from build123d import *

# Parameters (mm, degrees)
F0_R     = 5.08
F1_DEPTH = 91.44
F2_R     = 0.99
F3_DEPTH = 88.9
F4_SIZE  = 2.54
F5_R     = 5.08


with BuildPart() as f1:
    # F0 (on Front) → F1 (new body)
    with BuildSketch(Plane.XZ):
        Circle(F0_R)
    extrude(amount=F1_DEPTH)

    # F2 (on face) → F3 (cut)
    with BuildSketch(Plane.XZ.offset(91.44)):
        Circle(F2_R)
    extrude(amount=-F3_DEPTH, mode=Mode.SUBTRACT)

    # F4
    f4_edges = [f1.edges().sort_by_distance(p)[0] for p in [
        (-5.08, -91.44, 0),
    ]]
    chamfer(f4_edges, length=F4_SIZE)

    # F5
    f5_edges = [f1.edges().sort_by_distance(p)[0] for p in [
        (-5.08, 0, 0),
    ]]
    fillet(f5_edges, radius=F5_R)


solid = f1.part
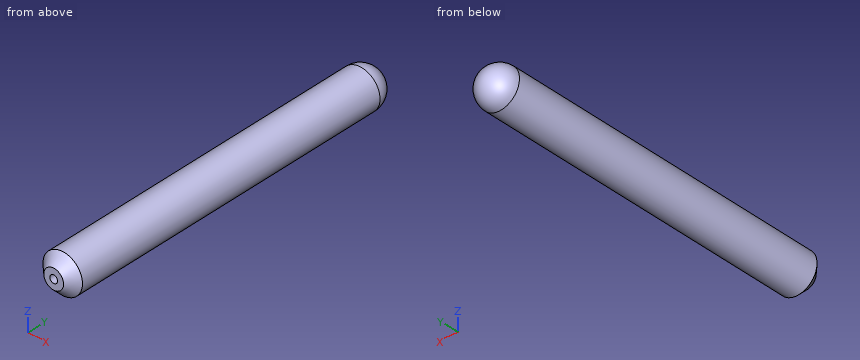
The listing builds one solid part. Answer for the finished solid, in the listing's coordinates (mm). Give positions to 0.01 mm unless a question says otherwise; leave off trailing zeros. Write each loop counter-clockwise with the first axis right and the second up, starting at its lowest first coordinate (ties: lowest second). Pieces come first, ordered by that corner, then holes. Notation, with made-up numbers: (-19.75, -16) -> (28.25, -16) arc R22 cw to (28.25, 17) -> close; hole circle Ø3 at (22.5, -24). An arc over 180 degrees is marked (long way). Use a Markdown table: item, result.
(1) Section A-A, the plane x = 0 is taken. Determine the outline of the cut face in (y, z).
Return value:
| item | result |
|---|---|
| outline | (-91.44, -2.54) -> (-88.9, -5.08) -> (-5.08, -5.08) arc R5.08 ccw to (-5.08, 5.08) -> (-88.9, 5.08) -> (-91.44, 2.54) -> (-91.44, 0.99) -> (-2.54, 0.99) -> (-2.54, -0.99) -> (-91.44, -0.99) -> close |
(2) Flat-ended cylindrical pins translate along their axes: P1, Ø1.5, axis at x = 3.5, y = -51.5, coming from the -Z side; P2, Ø1, axis at x = -2, y = -13.5, coming from the -Z side; P3, Ø3, axis at y = -61, z = -3.5, coming from the -X side. Find the tip coordinate at first contact, or state that the pin passes through.
Return value:
| item | result |
|---|---|
| P1 | z = -4.27 |
| P2 | z = -4.85 |
| P3 | x = -4.67 |
(3) Section B-B, the plane z = 0 is taken. Determine the outline of the cut face in (x, y).
Return value:
| item | result |
|---|---|
| outline | (-5.08, -88.9) -> (-2.54, -91.44) -> (-0.99, -91.44) -> (-0.99, -2.54) -> (0.99, -2.54) -> (0.99, -91.44) -> (2.54, -91.44) -> (5.08, -88.9) -> (5.08, -5.08) arc R5.08 ccw to (-5.08, -5.08) -> close |
(4) Section C-C, the plane y = -77.5 is taken. Determine the outline of the cut face in (x, z), then the cut area to 3 significant figures.
Return value:
| item | result |
|---|---|
| outline | circle Ø10.16 at (0, 0); hole circle Ø1.98 at (0, 0) |
| area | 78.0 mm2 |
(5) Find the intervals of material crossed by probe 1 along Z at (x, y) = (0, -59); probe 2 along Z at (x, y) = (0.75, -17); probe 3 along X at (y, z) = (-15, 0.5), in increasing order. Write a range as from..to.
Return value:
| item | result |
|---|---|
| probe 1 | -5.08..-0.99, 0.99..5.08 |
| probe 2 | -5.02..-0.65, 0.65..5.02 |
| probe 3 | -5.06..-0.85, 0.85..5.06 |
